from build123d import *

# Parameters (mm, degrees)
F1_DEPTH = 31.7246
F2_DEPTH = 16.51
F4_DEPTH = 6.35
F6_DEPTH = 16.51


with BuildPart() as f1:
    # F0 (on Top) → F1 (new body)
    with BuildSketch(Plane.XY):
        with BuildLine():
            ThreePointArc((26.2763, 3.2258), (24.654492, 7.141192), (20.7391, 8.763))
            Line((20.7391, 8.763), (-20.7391, 8.763))
            ThreePointArc((-20.7391, 8.763), (-23.251486, 8.16022), (-25.216874, 6.483118))
            Line((-25.216874, 6.483118), (-33.143533, 6.483118))
            ThreePointArc((-33.143533, 6.483118), (-37.002563, 4.916872), (-38.678471, 1.104186))
            Line((-38.678471, 1.104186), (-38.679923, 1.053386))
            ThreePointArc((-38.679923, 1.053386), (-37.115939, -2.963912), (-33.144986, -4.642082))
            Line((-33.144986, -4.642082), (-26.368298, -4.642082))
            ThreePointArc((-26.368298, -4.642082), (-24.393034, -7.613443), (-21.015287, -8.763))
            Line((-21.015287, -8.763), (20.7391, -8.763))
            ThreePointArc((20.7391, -8.763), (24.654492, -7.141192), (26.2763, -3.2258))
            Line((26.2763, -3.2258), (26.2763, 3.2258))
        make_face()
    extrude(amount=-F1_DEPTH)

    # F0 (on Top) → F2 (join)
    with BuildSketch(Plane.XY):
        with BuildLine():
            ThreePointArc((-38.678471, 1.104186), (-37.002563, 4.916872), (-33.143533, 6.483118))
            Line((-33.143533, 6.483118), (-38.910577, 6.483118))
            Line((-38.910577, 6.483118), (-57.0865, 6.483118))
            ThreePointArc((-57.0865, 6.483118), (-61.001892, 4.86131), (-62.6237, 0.945918))
            Line((-62.6237, 0.945918), (-62.6237, 0.895118))
            ThreePointArc((-62.6237, 0.895118), (-61.001892, -3.020274), (-57.0865, -4.642082))
            Line((-57.0865, -4.642082), (-38.839698, -4.642082))
            Line((-38.839698, -4.642082), (-33.144986, -4.642082))
            ThreePointArc((-33.144986, -4.642082), (-37.115939, -2.963912), (-38.679923, 1.053386))
            Line((-38.679923, 1.053386), (-38.678471, 1.104186))
        make_face()
    extrude(amount=-F2_DEPTH)

    # F3 (on face) → F4 (join)
    with BuildSketch(Plane(origin=(0, 0, -31.7246), x_dir=(1, 0, 0), z_dir=(0, 0, -1))):
        with BuildLine():
            ThreePointArc((-1.9939, 3.9624), (-5.9563, 0), (-1.9939, -3.9624))
            Line((-1.9939, -3.9624), (9.4361, -3.9624))
            ThreePointArc((9.4361, -3.9624), (13.3985, 0), (9.4361, 3.9624))
            Line((9.4361, 3.9624), (-1.9939, 3.9624))
        make_face()
    extrude(amount=F4_DEPTH)

    # F5 (on Top) → F6 (join)
    with BuildSketch(Plane.XY):
        with BuildLine():
            ThreePointArc((-57.0865, 6.483118), (-61.87738, 4.616227), (-64.141945, 0))
            ThreePointArc((-64.141945, 0), (-61.788333, -4.440921), (-57.0865, -6.216882))
            Line((-57.0865, -6.216882), (-38.839698, -6.216882))
            Line((-38.839698, -6.216882), (-38.839698, -4.598211))
            Line((-38.839698, -4.598211), (-38.839698, 6.483118))
            Line((-38.839698, 6.483118), (-57.0865, 6.483118))
        make_face()
    extrude(amount=-F6_DEPTH)


solid = f1.part
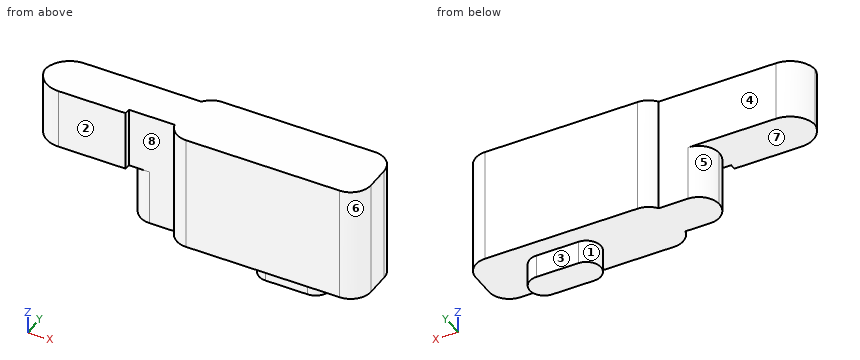
Work out the finished part from the listing and answer in its coordinate system (mm). Face numbers are marked on the shaded views. A direction names the side the tool comes from. Round coordinates to 2 decimals unless told otherwise and drop trailing zeros. Write each loop counter-clockwise with the first axis right and the second up, starting at its lowest first coordinate (ties: lowest second). Pieces come first, ordered by that corner, then holes. Notation, with made-up numbers: (46, 58) - (50, 58) arc R33 cw to (50, 93) - close; hole circle Ø11 at (60, 35.5). An arc over 180 degrees is marked (long way). Answer in a Markdown table with one row per item. Add a question column.
1. A cutting plane is placed at D-D, the plane z = -18. Determine the outline of the cut face in (x, y), and give its area (3 significant figures).
2. For the marked faces 1, 2, 3, 4 and 5, determine the directions among +Z, -Z, +X, -X, +Y, -Y from which every point of the face is accessible in a straight line to the end or side of a thin tool.
3. The mould has two halves that part along X. Classify the marked faces 6, 7 and 8: +X half, -X half, draft (parallel to the pull), parting line (faces both ways), or undercut.
4. A cutting plane is placed at C-C, the plane y = 5.25. Determine the outline of the cut face in (x, z).
5. A cutting plane is placed at B-B, the plane x = 5. Determine the outline of the cut face in (y, z), and give its area (3 significant figures).
6. A cutting plane is placed at A-A, the plane z = -8. Determine the outline of the cut face in (x, y), and give its area (3 significant figures).
7. Find the intervals of material crossed by line 1 along Z through (x, y) = (-27, 0.75); line 2 along Y through (x, z) = (-48.5, -5); line 3 along Z through (x, y) = (-43, -0.25), in increasing order. Write a range as from..to.
8. Given pin 1 (9.5 mm diameter, centred on x = -42.5, z = -22, fed in from +Y); pin 2 (4 mm diameter, centred on x = -41, z = -4, fed in from -Y); pin 3 (4 mm diameter, centred on x = -30, y = 3.5, fed in from -Z), each flat-ended and moving along its own axis, determine where each tip first touches the part or whether it passes through.
Worked out:
| question | item | result |
|---|---|---|
| 1 | outline | (-38.68, 1.05) arc R5.54 ccw to (-33.14, -4.64) - (-26.37, -4.64) arc R5.54 ccw to (-21.02, -8.76) - (20.74, -8.76) arc R5.54 ccw to (26.28, -3.23) - (26.28, 3.23) arc R5.54 ccw to (20.74, 8.76) - (-20.74, 8.76) arc R5.54 ccw to (-25.22, 6.48) - (-33.14, 6.48) arc R5.54 ccw to (-38.68, 1.1) - close |
| 1 | area | 1,020 mm^2 |
| 2 | face 1 | -Z, -X |
| 2 | face 2 | +Z, -Z, -X, -Y |
| 2 | face 3 | -Z, +X, -X, +Y |
| 2 | face 4 | +Z, -Z, -X, +Y |
| 2 | face 5 | -Z, -X, +Y |
| 3 | face 6 | +X half |
| 3 | face 7 | draft |
| 3 | face 8 | undercut |
| 4 | outline | (-61.08, -16.51) - (-36.63, -16.51) - (-36.63, -31.72) - (25.89, -31.72) - (25.89, 0) - (-61.08, 0) - close |
| 5 | outline | (-8.76, -31.72) - (-3.96, -31.72) - (-3.96, -38.07) - (3.96, -38.07) - (3.96, -31.72) - (8.76, -31.72) - (8.76, 0) - (-8.76, 0) - close |
| 5 | area | 606 mm^2 |
| 6 | outline | (-64.14, 0) arc R7.11 ccw to (-57.09, -6.22) - (-38.84, -6.22) - (-38.84, -4.64) - (-26.37, -4.64) arc R5.54 ccw to (-21.02, -8.76) - (20.74, -8.76) arc R5.54 ccw to (26.28, -3.23) - (26.28, 3.23) arc R5.54 ccw to (20.74, 8.76) - (-20.74, 8.76) arc R5.54 ccw to (-25.22, 6.48) - (-57.09, 6.48) arc R7.08 ccw to start |
| 6 | area | 1,340 mm^2 |
| 7 | line 1 | -31.72..0 |
| 7 | line 2 | -6.22..6.48 |
| 7 | line 3 | -16.51..0 |
| 8 | pin 1 | y = 4.02 |
| 8 | pin 2 | y = -6.22 |
| 8 | pin 3 | z = -31.72 |
